```python
from build123d import *

# Parameters (mm, degrees)
SKETCH1_W           = 25.4
SKETCH1_H           = 12.7
BOSS_EXTRUDE1_DEPTH = 2.54
SKETCH2_W           = 9.583787324
SKETCH2_H           = 9.041308796
SKETCH2_W_2         = 8.602159512
SKETCH2_H_2         = 3.926511249
BOSS_EXTRUDE2_DEPTH = 1.27
SKETCH3_W           = 5.506895622
SKETCH3_H           = 5.893999151
SKETCH3_W_2         = 1.890426858
SKETCH3_H_2         = 2.97685463
SKETCH3_H_3         = 2.926527621
SKETCH3_H_4         = 2.612813109
SKETCH3_W_3         = 5.17306174
SKETCH3_H_5         = 3.865660491
BOSS_EXTRUDE3_DEPTH = 1.27


with BuildPart() as part:
    # Sketch1 → Boss-Extrude1 (new body)
    with BuildSketch(Plane(origin=(0, 0, 0), x_dir=(1, 0, 0), z_dir=(0, 1, 0))):
        Rectangle(SKETCH1_W, SKETCH1_H)
    extrude(amount=BOSS_EXTRUDE1_DEPTH)

    # Sketch2 → Boss-Extrude2 (add)
    with BuildSketch(Plane(origin=(0, 2.54, 0), x_dir=(1, 0, 0), z_dir=(0, 1, 0))):
        with Locations((-6.26433538, 0.090413088)):
            Rectangle(SKETCH2_W, SKETCH2_H)
        with Locations((5.386036811, -2.311991821)):
            Rectangle(SKETCH2_W_2, SKETCH2_H_2)
    extrude(amount=BOSS_EXTRUDE2_DEPTH)

    # Sketch3 → Boss-Extrude3 (add)
    with BuildSketch(Plane.XZ):
        with Locations((-1.163587027, 0.709784011)):
            Rectangle(SKETCH3_W, SKETCH3_H)
        with Locations((-10.984373833, -3.72564288)):
            Rectangle(SKETCH3_W_2, SKETCH3_H_2)
        with Locations((-10.984373833, 0.369096396)):
            Rectangle(SKETCH3_W_2, SKETCH3_H_3)
        with Locations((-10.984373833, 4.175284666)):
            Rectangle(SKETCH3_W_2, SKETCH3_H_4)
        with Locations((6.004852016, 3.317890469)):
            Rectangle(SKETCH3_W_3, SKETCH3_H_5)
    extrude(amount=BOSS_EXTRUDE3_DEPTH)


solid = part.part
```
Input: part model. Units: mm. Frame: model coordinates. A direction names the side the tool comes from. Round coordinates to 2 decimals unless told otherwise and drop trailing zeros. Order: outer loops, then holes, each group sorted by start corner. A loop starts at its lowest first (then second) coordinate and runs counter-clockwise, first axis right, second up. Notation, with made-up numbers: (21, 81) - (41, 81) arc R27 ccw to (41, 107) - close; hole circle Ø8 at (-36.75, -20). An arc over 180 degrees is marked (long way). Answer in a Markdown table with one row per item.
Item 1: Reachability of faces 1 (the flat face through (-11.056, 3, 0)), 2 (the flat face through (1.085, 3, 2)), 3 (the flat face through (-11, -1, 5.482)), 4 (the flat face through (6, -1, 1.385)) from +Z, -Z, +X, -X, +Y, -Y: full face, straight path, thin tool, end or side. Return the list, or none.
Model answer:
| item | result |
|---|---|
| face 1 | +Z, -Z, -X, +Y |
| face 2 | +Z, -Z, +Y |
| face 3 | +Z, +X, -X, -Y |
| face 4 | -Z, +X, -Y |
Item 2: Pin query (flat end, axial travel): pin 1 (0.6 mm diameter, centred on y = 3.5, z = 3, fed in from +X); pin 2 (2 mm diameter, centred on x = 6.5, z = -4.5, fed in from -Y); pin 3 (1 mm diameter, centred on y = -1, z = 2, fed in from +X). Return the tip coordinate at first contact, or that it passes through.
Model answer:
| item | result |
|---|---|
| pin 1 | stops at x = 9.69 |
| pin 2 | stops at y = 0 |
| pin 3 | stops at x = 8.59 |
Item 3: Line query: line 1 (X direction, y = -0.05, z = 3.5); line 2 (X direction, y = -0.25, z = -0.75); line 3 (Y direction, x = 10, z = 1). Output: solid intervals per line, ascending.
Model answer:
| item | result |
|---|---|
| line 1 | x = -11.93 to -10.04, -3.92 to 1.59, 3.42 to 8.59 |
| line 2 | x = -11.93 to -10.04, -3.92 to 1.59 |
| line 3 | y = 0 to 2.54 |
Item 4: Section query A-A (y = 3.35). Return the cut outline in (x, z).
Model answer:
| item | result |
|---|---|
| outline | (-11.06, -4.61) - (-1.47, -4.61) - (-1.47, 4.43) - (-11.06, 4.43) - close; (1.08, 0.35) - (9.69, 0.35) - (9.69, 4.28) - (1.08, 4.28) - close |
Item 5: Section query D-D (x = 4). Return the cut outline in (y, z), then the cut area to 3 significant figures.
Model answer:
| item | result |
|---|---|
| outline | (-1.27, 1.39) - (0, 1.39) - (0, -6.35) - (2.54, -6.35) - (2.54, 0.35) - (3.81, 0.35) - (3.81, 4.28) - (2.54, 4.28) - (2.54, 6.35) - (0, 6.35) - (0, 5.25) - (-1.27, 5.25) - close |
| area | 42.2 mm² |
Item 6: Section query B-B (z = -3.5). Return the cut outline in (x, y), then the cut area to 3 significant figures.
Model answer:
| item | result |
|---|---|
| outline | (-12.7, 0) - (-11.93, 0) - (-11.93, -1.27) - (-10.04, -1.27) - (-10.04, 0) - (12.7, 0) - (12.7, 2.54) - (-1.47, 2.54) - (-1.47, 3.81) - (-11.06, 3.81) - (-11.06, 2.54) - (-12.7, 2.54) - close |
| area | 79.1 mm² |
Item 7: Section query C-C (x = 0.5). Return the cut outline in (y, z), then the cut area to 3 significant figures.
Model answer:
| item | result |
|---|---|
| outline | (-1.27, -2.24) - (0, -2.24) - (0, -6.35) - (2.54, -6.35) - (2.54, 6.35) - (0, 6.35) - (0, 3.66) - (-1.27, 3.66) - close |
| area | 39.7 mm² |
Item 8: Mould query, pull axis Z, two halves, no side actions, for faces 5 (the flat face through (-11, -1, -1.094)), 6 (the flat face through (-1, -1, -2.237)), 7 (the flat face through (3.418, -1, 3)). Classes: released by +Z, released by -Z, zero draft, split by the parting line, or undercut.
Model answer:
| item | result |
|---|---|
| face 5 | undercut |
| face 6 | released by -Z |
| face 7 | zero draft |
